from build123d import *

# Parameters (mm, degrees)
F0_W     = 101.6
F0_H     = 69.85
F0_W_2   = 38.1
F0_H_2   = 17.780002
F1_DEPTH = 25.4
F2_R     = 10.192823
F3_DEPTH = 50.801
F4_R     = 12.7


with BuildPart() as f1:
    # F0 (on Front) → F1 (new body, symmetric)
    with BuildSketch(Plane.XZ):
        Rectangle(F0_W, F0_H)
        Rectangle(F0_W_2, F0_H_2, mode=Mode.SUBTRACT)
    extrude(amount=F1_DEPTH, both=True)

    # F2 (on face) → F3 (cut, through all)
    with BuildSketch(Plane.XZ.offset(25.4)):
        with Locations((33.223767, 0)):
            Circle(F2_R)
    extrude(amount=-F3_DEPTH, mode=Mode.SUBTRACT)

    # F4
    f4_edges = [f1.edges().sort_by_distance(p)[0] for p in [
        (-50.8, 0, 34.925),
        (50.8, 0, 34.925),
        (50.8, 0, -34.925),
        (-50.8, 0, -34.925),
    ]]
    fillet(f4_edges, radius=F4_R)


solid = f1.part
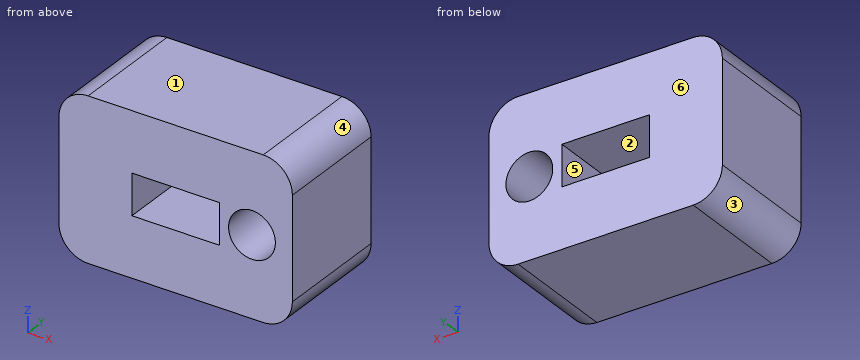
Can you work these out from the model? Positions are in its coordinate system, mm. Face numbers are marked on the shaded views. A direction names the side the tool comes from. Round coordinates to 2 decimals unless told otherwise and drop trailing zeros. Loops run counter-clockwise (first coordinate to the right, second up) from the corner with the lowest first, then second, coordinate; pieces in that order, holes last. Notation, with made-up numbers: (65, -31) - (93, -31) arc R8 cw to (93, -18) - close; hole circle Ø7 at (59, 39). An arc over 180 degrees is marked (long way). Use CSV: the item, a comma, the result in double quotes. Start each with the question number.
1) If we section it at B-B on x = 32: Write out the boundary of the cut face in (y, z) (3 decimals).
2) Please list where these lines run through material, in increasing order: probe 1 along Z at (x, y) = (-5.5, -14) (3 decimals); probe 2 along X at (y, z) = (-3, 8); probe 3 along X at (y, z) = (-18, -3.5). Write a range as [from, to].
3) If we section it at C-C on y = 3.5: Write out the boundary of the cut face in (x, z) (3 decimals), plus the area to 3 significant figures.
4) We'd pull the mould along Z, two halves only. Please class the marked faces 3, 4, 5 and 6: released by +Z, released by -Z, zero draft, split by the parting line, or undercut.
5) If we section it at A-A on z = 0: Write out the boundary of the cut face in (x, y), plus the area to 3 significant figures.
6) For pin 1 Ø10 at (y, z) = (2, -23.5) entering from +X, with a flat end and sliding along its axis, tell me the tip position at first contact or that it passes through.
7) For the marked faces 1 and 2, which set-ups out of +Z, -Z, +X, -X, +Y, -Y let a thin tool reach every point of the face, with its end or its side?
8) If we section it at D-D on z = -30: Write out the boundary of the cut face in (x, y), plus the area to 3 significant figures.
Geometry results:
1,outline,"(-25.4, -34.925) - (25.4, -34.925) - (25.4, -10.119) - (-25.4, -10.119) - close; (-25.4, 10.119) - (25.4, 10.119) - (25.4, 34.925) - (-25.4, 34.925) - close"
2,probe 1,"z = [-34.925, -8.89], [8.89, 34.925]"
2,probe 2,"x = [-50.8, -19.05], [19.05, 26.91], [39.54, 50.8]"
2,probe 3,"x = [-50.8, -19.05], [19.05, 23.65], [42.8, 50.8]"
3,outline,"(-50.8, -22.225) arc R12.7 ccw to (-38.1, -34.925) - (38.1, -34.925) arc R12.7 ccw to (50.8, -22.225) - (50.8, 22.225) arc R12.7 ccw to (38.1, 34.925) - (-38.1, 34.925) arc R12.7 ccw to (-50.8, 22.225) - close; hole (-19.05, -8.89) - (19.05, -8.89) - (19.05, 8.89) - (-19.05, 8.89) - close; hole circle Ø20.386 at (33.224, 0)"
3,area,"5,950 mm2"
4,face 3,"released by -Z"
4,face 4,"released by +Z"
4,face 5,"undercut"
4,face 6,"zero draft"
5,outline,"(-50.8, -25.4) - (-19.05, -25.4) - (-19.05, 25.4) - (-50.8, 25.4) - close; (19.05, -25.4) - (23.03, -25.4) - (23.03, 25.4) - (19.05, 25.4) - close; (43.42, -25.4) - (50.8, -25.4) - (50.8, 25.4) - (43.42, 25.4) - close"
5,area,"2,190 mm2"
6,pin 1,"stops at x = 50.8"
7,face 1,"+Z, +X, -X, +Y, -Y"
7,face 2,"+Y, -Y"
8,outline,"(-48.14, -25.4) - (48.14, -25.4) - (48.14, 25.4) - (-48.14, 25.4) - close"
8,area,"4,890 mm2"
